Input: part model. Units: mm. Frame: model coordinates. Face numbers are marked on the shaded views. A direction names the side the tool comes from. Round coordinates to 2 decimals unless told otherwise and drop trailing zeros. Loops run counter-clockwise (first coordinate to the right, second up) from the corner with the lowest first, then second, coordinate; pieces in that order, holes last. Notation, with made-up numbers: (-11.75, -13) -> (-4.75, -13) arc R23 ccw to (-4.75, 15) -> close; hole circle Ø1 at (-22.5, -38). An arc over 180 degrees is marked (long way). Answer in a Markdown table with one row per item. Add a question column.
Q1. Section A-A, the plane y = 0. Output: boundary loops of the cut face in (x, z), and give its area (3 significant figures).
Q2. Mould query, pull axis Z, two halves, no side actions, for the marked faces 3, 4 and 5. Classes: pulls with the +Z half, pulls with the -Z half, needs draft (parallel to the pull), parting line crosses it, or undercut.
Q3. Reachability of the marked faces 1 and 2 from +Z, -Z, +X, -X, +Y, -Y: full face, straight path, thin tool, end or side. Return the list, or none.
Q4. Section C-C, the plane z = -8.75. Output: boundary loops of the cut face in (x, y), and give its area (3 significant figures).
Q5. Section B-B, the plane x = 0. Output: boundary loops of the cut face in (y, z).
Q6. Section D-D, the plane x = -16.5. Output: boundary loops of the cut face in (y, z), and give its area (3 significant figures).
Q7. Pin query (flat end, axial travel): pin 1 (3 mm diameter, centred on y = 8, z = -11, fed in from -X); pin 2 (5 mm diameter, centred on y = 12.5, z = -4.5, fed in from +X); pin 3 (3 mm diameter, centred on x = 10.5, z = -9.5, fed in from -Y); pin 4 (3 mm diameter, centred on x = 0, z = -10, fed in from +Y). Return the tip coordinate at first contact, or that it passes through.
Q8. Ray query, L1, parallel to Y at x = 0, z = -11.9; L2, parallel to Y at x = 0, z = -6.5; L3, parallel to Y at x = 1, z = -13.75. Return the intervals inside material, ascending. Write a range as from..to.
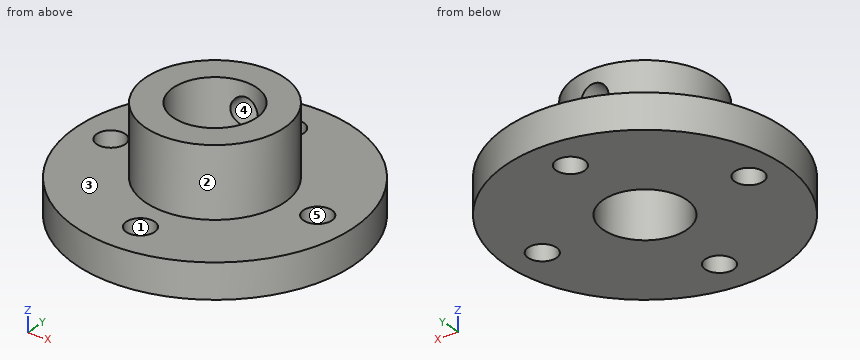
```python
from build123d import *

# Parameters (mm, degrees)
F2_R     = 6
F3_DEPTH = 45
F4_R     = 2.05
F5_DEPTH = 25
F6_R     = 2
F7_DEPTH = 10


with BuildPart() as f1:
    # F0 (on Front) → F1 (revolve)
    with BuildSketch(Plane.XZ):
        Polygon((0, -15), (0, 0), (-10, 0), (-10, -10), (-20, -10), (-20, -15), align=None)
    revolve(axis=Axis((0, 0, -7.5), (0, 0, -1)))

    # F2 (on face) → F3 (cut)
    with BuildSketch(Plane.XY):
        Circle(F2_R)
    extrude(amount=-F3_DEPTH, mode=Mode.SUBTRACT)

    # F4 (on Top) → F5 (cut)
    with BuildSketch(Plane.XY):
        with Locations((0, 14.49627)):
            Circle(F4_R)
        with Locations((0, -14.49627)):
            Circle(F4_R)
        with Locations((14.88806, 0)):
            Circle(F4_R)
        with Locations((-15.083956, 0)):
            Circle(F4_R)
    extrude(amount=-F5_DEPTH, mode=Mode.SUBTRACT)

    # F6 (on Front) → F7 (cut)
    with BuildSketch(Plane.XZ):
        with Locations((0, -4)):
            Circle(F6_R)
    extrude(amount=-F7_DEPTH, mode=Mode.SUBTRACT)


solid = f1.part
```
Answer block:
| question | item | result |
|---|---|---|
| 1 | outline | (-20, -15) -> (-17.13, -15) -> (-17.13, -10) -> (-20, -10) -> close; (-13.03, -15) -> (-6, -15) -> (-6, 0) -> (-10, 0) -> (-10, -10) -> (-13.03, -10) -> close; (6, -15) -> (12.84, -15) -> (12.84, -10) -> (10, -10) -> (10, 0) -> (6, 0) -> close; (16.94, -15) -> (20, -15) -> (20, -10) -> (16.94, -10) -> close |
| 1 | area | 179 mm^2 |
| 2 | face 3 | pulls with the +Z half |
| 2 | face 4 | undercut |
| 2 | face 5 | needs draft |
| 3 | face 1 | +Z, -Z |
| 3 | face 2 | +Z |
| 4 | outline | circle Ø20 at (0, 0); hole circle Ø12 at (0, 0) |
| 4 | area | 201 mm^2 |
| 5 | outline | (-20, -15) -> (-16.55, -15) -> (-16.55, -10) -> (-20, -10) -> close; (-12.45, -15) -> (-6, -15) -> (-6, 0) -> (-10, 0) -> (-10, -10) -> (-12.45, -10) -> close; (6, -15) -> (12.45, -15) -> (12.45, -10) -> (10, -10) -> (10, -6) -> (6, -6) -> close; (6, -2) -> (10, -2) -> (10, 0) -> (6, 0) -> close; (16.55, -15) -> (20, -15) -> (20, -10) -> (16.55, -10) -> close |
| 6 | outline | (-11.3, -15) -> (-1.48, -15) -> (-1.48, -10) -> (-11.3, -10) -> close; (1.48, -15) -> (11.3, -15) -> (11.3, -10) -> (1.48, -10) -> close |
| 6 | area | 98.2 mm^2 |
| 7 | pin 1 | x = -18.91 |
| 7 | pin 2 | through |
| 7 | pin 3 | y = -17.82 |
| 7 | pin 4 | y = 20 |
| 8 | L1 | -20..-16.55, -12.45..-6, 6..12.45, 16.55..20 |
| 8 | L2 | -10..-6, 6..10 |
| 8 | L3 | -19.97..-16.29, -12.71..-5.92, 5.92..12.71, 16.29..19.97 |
